Job drawing, mm, ordinate dimensions from the low corner. One solid piece. Give positions to 0.01 mm unless a question says otherwise; leave off trailing zeros. Loops run counter-clockwise (first coordinate to the right, second up) from the corner with the lowest first, then second, coordinate; pieces in that order, holes last. Notation, with made-up numbers: (51.25, 14) - (86.25, 14) arc R17 cw to (86.25, 38) - close; hole circle Ø2 at (53.5, 17). An arc over 180 degrees is marked (long way). Use a Markdown table: item, result.
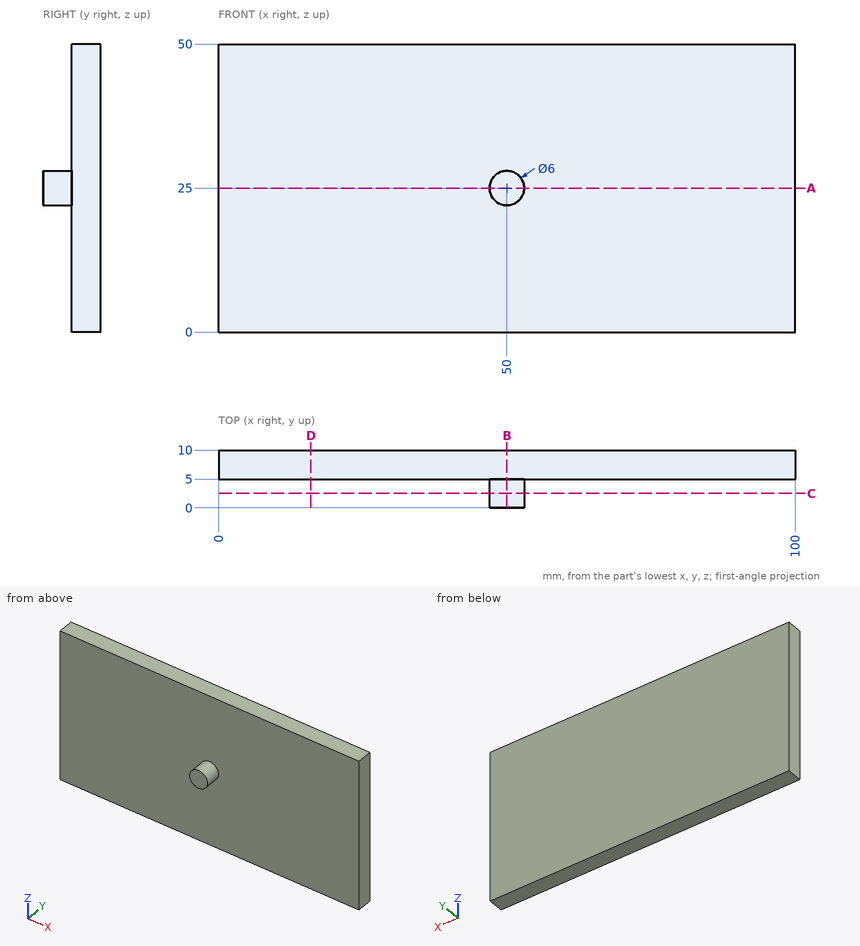
(1) Slice it at A-A, the plane z = 25. Write the cut outline in (x, y), plus the area to 3 significant figures.
Computed:
| item | result |
|---|---|
| outline | (0, 5) - (47, 5) - (47, 0) - (53, 0) - (53, 5) - (100, 5) - (100, 10) - (0, 10) - close |
| area | 530 mm² |
(2) Slice it at D-D, the plane x = 16. Write the cut outline in (y, z), plus the area to 3 significant figures.
Computed:
| item | result |
|---|---|
| outline | (5, 0) - (10, 0) - (10, 50) - (5, 50) - close |
| area | 250 mm² |
(3) Slice it at B-B, the plane x = 50. Write the cut outline in (y, z).
Computed:
| item | result |
|---|---|
| outline | (0, 22) - (5, 22) - (5, 0) - (10, 0) - (10, 50) - (5, 50) - (5, 28) - (0, 28) - close |
(4) Slice it at C-C, the plane y = 2.5. Write the cut outline in (x, z).
Computed:
| item | result |
|---|---|
| outline | circle Ø6 at (50, 25) |
(5) Pin check, flat tip, straight feed: P1, Ø10, axis at x = 36, z = 23.5, coming from the -Y side. Stop position of the tip, or through.
Computed:
| item | result |
|---|---|
| P1 | y = 5 |
(6) Drill centre lines: probe 1 along Y at (x, z) = (39.5, 3); probe 2 along X at (y, z) = (4.75, 25.5). Where is each one in solid material? Low to high. Write a range as [from, to].
Computed:
| item | result |
|---|---|
| probe 1 | [5, 10] |
| probe 2 | [47.04, 52.96] |
